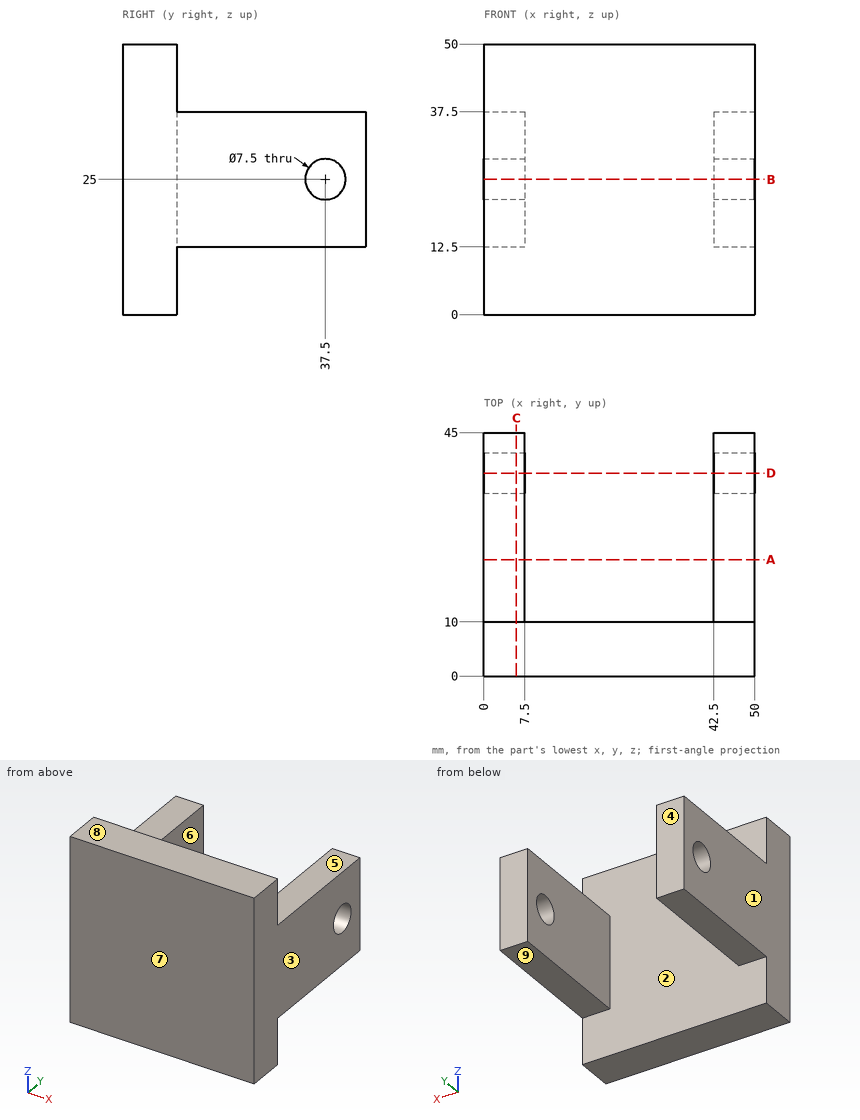
Geometry check sheet. Reference: drawing and pictorial views, mm from the part's lowest x, y, z. A direction names the side the tool comes from. Coordinates: 2 decimals unless noted, no trailing zeros. Loops run counter-clockwise (first coordinate to the right, second up) from the corner with the lowest first, then second, coordinate; pieces in that order, holes last. Notation, with made-up numbers: (-27, 69.5) - (2, 69.5) arc R25 ccw to (2, 107.5) - close; hole circle Ø5 at (83, 0.25). An arc over 180 degrees is marked (long way). Return JSON: item names as keys, results as strings.
1. Section check A-A, the plane y = 21.5. Record the boundary of the cut face in (x, z).
Established:
{"outline": "(0, 12.5) - (7.5, 12.5) - (7.5, 37.5) - (0, 37.5) - close; (42.5, 12.5) - (50, 12.5) - (50, 37.5) - (42.5, 37.5) - close"}
2. Tool access check on the marked faces 5, 6, 7, 8 and 9. Record the directions out of +Z, -Z, +X, -X, +Y, -Y that give a thin tool (end or side, any length) a straight path to the whole face; none if there is none.
Established:
{"face 5": "+Z, +X, -X, +Y", "face 6": "+Z, -Z, +Y", "face 7": "+Z, -Z, +X, -X, -Y", "face 8": "+Z, +X, -X, +Y, -Y", "face 9": "-Z, +X, -X, +Y"}
3. Section check C-C, the plane x = 6. Record the boundary of the cut face in (y, z), then the cut area to 3 significant figures.
Established:
{"outline": "(0, 0) - (10, 0) - (10, 12.5) - (45, 12.5) - (45, 37.5) - (10, 37.5) - (10, 50) - (0, 50) - close; hole circle Ø7.5 at (37.5, 25)", "area": "1,330 mm2"}
4. Section check D-D, the plane y = 37.5. Record the boundary of the cut face in (x, z), then the cut area to 4 significant figures.
Established:
{"outline": "(0, 12.5) - (7.5, 12.5) - (7.5, 21.25) - (0, 21.25) - close; (0, 28.75) - (7.5, 28.75) - (7.5, 37.5) - (0, 37.5) - close; (42.5, 12.5) - (50, 12.5) - (50, 21.25) - (42.5, 21.25) - close; (42.5, 28.75) - (50, 28.75) - (50, 37.5) - (42.5, 37.5) - close", "area": "262.5 mm2"}
5. Section check B-B, the plane z = 25. Record the boundary of the cut face in (x, y).
Established:
{"outline": "(0, 0) - (50, 0) - (50, 33.75) - (42.5, 33.75) - (42.5, 10) - (7.5, 10) - (7.5, 33.75) - (0, 33.75) - close; (0, 41.25) - (7.5, 41.25) - (7.5, 45) - (0, 45) - close; (42.5, 41.25) - (50, 41.25) - (50, 45) - (42.5, 45) - close"}
6. Thickness scan on L1, parallel to Y at x = 4, z = 25; L2, parallel to X at y = 34.5, z = 36; L3, parallel to Y at x = 25.5, z = 39. Record the ranges inside material, lowest first.
Established:
{"L1": "y = 0 to 33.75, 41.25 to 45", "L2": "x = 0 to 7.5, 42.5 to 50", "L3": "y = 0 to 10"}
7. Mould release check, pull along X, two halves, no side actions. Record for the marked faces 1, 2, 3 and 4: +X half, -X half, draft (parallel to the pull), parting line (faces both ways), or undercut.
Established:
{"face 1": "-X half", "face 2": "undercut", "face 3": "+X half", "face 4": "draft"}
8. Go/stop test with flat-tipped pins: pin 1 (2 mm diameter, centred on x = 46.5, y = 28, fed in from -Z); pin 2 (4 mm diameter, centred on x = 47.5, y = 23, fed in from +Z); pin 3 (10 mm diameter, centred on x = 24, z = 38, fed in from +Y). Record where each tip stops, or that it passes through.
Established:
{"pin 1": "stops at z = 12.5", "pin 2": "stops at z = 37.5", "pin 3": "stops at y = 10"}
